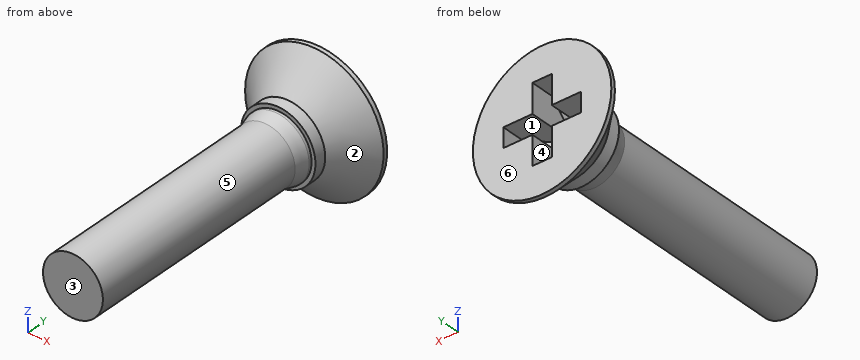
from build123d import *

# Parameters (mm, degrees)
KREUZSCHLITZ1_H_DEPTH      = 0.65
KREUZSCHLITZ1_H_DEPTH_BACK = 0.65
KREUZSCHLITZ2_H_DEPTH      = 0.65
KREUZSCHLITZ2_H_DEPTH_BACK = 0.65
BOSS_EXTRUDE1_START        = 4
SKETCH1_R                  = 2.0095
BOSS_EXTRUDE1_DEPTH        = 4


with BuildPart() as part:
    # Skizze1 → Basis-Rotation (revolve)
    with BuildSketch(Plane.XY, mode=Mode.PRIVATE) as basis_rotation_sk:
        Polygon((0, 0), (4.65, 0), (4.65, -0.29), (2.5, -2.44), (2.5, -3.24), (2.24, -3.24), (2.24, -3.439762289), (2.0095, -4.3), (2.0095, -16), (0, -16), align=None)
    revolve(basis_rotation_sk.sketch.rotate(Axis((0, 0, 0), (0, -1, 0)), 180), axis=Axis((0, 0, 0), (0, -1, 0)))

    # Skizze2 → Kreuzschlitz1 H (cut, two sides: drawn at the far end of the back side and taken through both)
    with BuildSketch(Plane.XY.offset(-KREUZSCHLITZ1_H_DEPTH_BACK)):
        Polygon((-1, -3.2), (1, -3.2), (2.6, -1.6), (2.6, 0), (-2.6, 0), (-2.6, -1.6), align=None)
    extrude(amount=KREUZSCHLITZ1_H_DEPTH + KREUZSCHLITZ1_H_DEPTH_BACK, mode=Mode.SUBTRACT)

    # Skizze3 → Kreuzschlitz2 H (cut, two sides: drawn at the far end of the back side and taken through both)
    with BuildSketch(Plane(origin=(0, 0, 0), x_dir=(0, 0, -1), z_dir=(1, 0, 0)).offset(-KREUZSCHLITZ2_H_DEPTH_BACK)):
        Polygon((-1, -3.2), (1, -3.2), (2.6, -1.6), (2.6, 0), (-2.6, 0), (-2.6, -1.6), align=None)
    extrude(amount=KREUZSCHLITZ2_H_DEPTH + KREUZSCHLITZ2_H_DEPTH_BACK, mode=Mode.SUBTRACT)

    # Sketch1 → Boss-Extrude1 (add)
    with BuildSketch(Plane.XZ.offset(16).offset(BOSS_EXTRUDE1_START)):
        with Locations(Location((0, 0, 0), (0, 0, 180))):
            Circle(SKETCH1_R)
    extrude(amount=-BOSS_EXTRUDE1_DEPTH)


solid = part.part
Geometry check sheet. Reference: the model listing, model coordinates, mm. Face numbers are marked on the shaded views. A direction names the side the tool comes from. Give positions to 0.01 mm unless a question says otherwise; leave off trailing zeros. Loops run counter-clockwise (first coordinate to the right, second up) from the corner with the lowest first, then second, coordinate; pieces in that order, holes last. Notation, with made-up numbers: M 61.25,18.5 L 118.25,18.5 A23 ccw 118.25,31.5 Z; hole C -24.5,23 d2. An arc over 180 degrees is marked long. Answer as a JSON object with one key per item and string values. Group by question number.
Item 1: Access from +Z, -Z, +X, -X, +Y, -Y to the whole of each face (thin tool, end or side, straight path). Record for the marked faces 4, 5 and 6.
Item 2: Sectioned sample at B-B on y = -7. Record the boundary of the cut face in (x, z), plus the area to 3 significant figures.
Item 3: Gauge pin test, flat ends, axial feed: pin 1 (5 mm diameter, centred on y = -4.5, z = 1.5, fed in from -X); pin 2 (2 mm diameter, centred on y = -1, z = 1.5, fed in from -X); pin 3 (1 mm diameter, centred on x = 1.5, y = -1.5, fed in from -Z). Record the tip position at first contact, or that the pin passes through.
Item 4: Mould release check, pull along X, two halves, no side actions. Record for the marked faces 1, 2 and 3: pulls with the +X half, pulls with the -X half, needs draft (parallel to the pull), parting line crosses it, or undercut.
Item 5: Sectioned sample at A-A on x = 0. Record the boundary of the cut face in (y, z).
Item 6: Material ranges on L1, parallel to Z at x = -0.5, y = -0.75; L2, parallel to Y at x = 0.25, z = -0.5; L3, parallel to X at y = -1.5, z = -2, recorded low to high.
Findings below:
{
 "1": {"face 4": "+Y", "face 5": "-Y", "face 6": "+Z, -Z, +X, -X, +Y"},
 "2": {"outline": "C 0,0 d4.02", "area": "12.7 mm2"},
 "3": {"pin 1": "x = -2.73", "pin 2": "x = -4.58", "pin 3": "z = -3.68"},
 "4": {"face 1": "undercut", "face 2": "parting line crosses it", "face 3": "needs draft"},
 "5": {"outline": "M -20,-2.01 L -4.3,-2.01 L -3.44,-2.24 L -3.24,-2.24 L -3.24,-2.5 L -2.44,-2.5 L -0.29,-4.65 L 0,-4.65 L 0,-2.6 L -1.6,-2.6 L -3.2,-1 L -3.2,1 L -1.6,2.6 L 0,2.6 L 0,4.65 L -0.29,4.65 L -2.44,2.5 L -3.24,2.5 L -3.24,2.24 L -3.44,2.24 L -4.3,2.01 L -20,2.01 Z"},
 "6": {"L1": "-4.16 to -2.6, 2.6 to 4.16", "L2": "-20 to -3.2", "L3": "-2.8 to -0.65, 0.65 to 2.8"}
}
